from build123d import *

# Parameters (mm, degrees)
SKETCH1_R           = 54
SKETCH1_R_2         = 41
BOSS_EXTRUDE1_DEPTH = 10
SKETCH2_R           = 4.1
CUT_EXTRUDE1_DEPTH  = 5
CUT_EXTRUDE2_REACH  = 78.531
SKETCH3_R           = 3.1
CHAMFER1_SIZE       = 1


with BuildPart() as part:
    # Sketch1 → Boss-Extrude1 (new body)
    with BuildSketch(Plane(origin=(0, 0, 0), x_dir=(1, 0, 0), z_dir=(0, 1, 0))):
        with Locations(Location((0, 0, 0), (0, 0, 270))):
            Circle(SKETCH1_R)
        with Locations(Location((0, 0, 0), (0, 0, 270))):
            Circle(SKETCH1_R_2, mode=Mode.SUBTRACT)
    extrude(amount=BOSS_EXTRUDE1_DEPTH)

    # Sketch2 → Cut-Extrude1 (cut)
    with BuildSketch(Plane(origin=(0, 10, 0), x_dir=(1, 0, 0), z_dir=(0, 1, 0))):
        with Locations(Location((0, 47.5, 0), (0, 0, 270))):
            Circle(SKETCH2_R)
        with Locations(Location((41.13620668, -23.75, 0), (0, 0, 270))):
            Circle(SKETCH2_R)
        with Locations(Location((-41.13620668, -23.75, 0), (0, 0, 270))):
            Circle(SKETCH2_R)
    extrude(amount=-CUT_EXTRUDE1_DEPTH, mode=Mode.SUBTRACT)

    # Sketch3 → Cut-Extrude2 (cut, up to next)
    with BuildSketch(Plane(origin=(0, 5, 0), x_dir=(1, 0, 0), z_dir=(0, 1, 0)), mode=Mode.PRIVATE) as cut_extrude2_sk1:
        with Locations(Location((0, 47.5, 0), (0, 0, 270))):
            Circle(SKETCH3_R)
    cut_extrude2_tool1 = extrude(cut_extrude2_sk1.sketch, amount=-CUT_EXTRUDE2_REACH, mode=Mode.PRIVATE) & part.part
    # Sketch3 → Cut-Extrude2 (cut, up to next)
    with BuildSketch(Plane(origin=(0, 5, 0), x_dir=(1, 0, 0), z_dir=(0, 1, 0)), mode=Mode.PRIVATE) as cut_extrude2_sk2:
        with Locations(Location((41.13620668, -23.75, 0), (0, 0, 270))):
            Circle(SKETCH3_R)
    cut_extrude2_tool2 = extrude(cut_extrude2_sk2.sketch, amount=-CUT_EXTRUDE2_REACH, mode=Mode.PRIVATE) & part.part
    # Sketch3 → Cut-Extrude2 (cut, up to next)
    with BuildSketch(Plane(origin=(0, 5, 0), x_dir=(1, 0, 0), z_dir=(0, 1, 0)), mode=Mode.PRIVATE) as cut_extrude2_sk3:
        with Locations(Location((-41.13620668, -23.75, 0), (0, 0, 270))):
            Circle(SKETCH3_R)
    cut_extrude2_tool3 = extrude(cut_extrude2_sk3.sketch, amount=-CUT_EXTRUDE2_REACH, mode=Mode.PRIVATE) & part.part
    add(cut_extrude2_tool1.solids().sort_by_distance((0, 5, -47.5))[0], mode=Mode.SUBTRACT)
    add(cut_extrude2_tool2.solids().sort_by_distance((41.136207, 5, 23.75))[0], mode=Mode.SUBTRACT)
    add(cut_extrude2_tool3.solids().sort_by_distance((-41.136207, 5, 23.75))[0], mode=Mode.SUBTRACT)

    # Chamfer1
    chamfer1_edges = [part.edges().sort_by_distance(p)[0] for p in [
        (0, 10, -51.6),
        (41.13620668, 10, 19.65),
        (-41.13620668, 10, 19.65),
    ]]
    chamfer(chamfer1_edges, length=CHAMFER1_SIZE)


solid = part.part
Read the model definition and answer for the solid it produces. Units are mm, in the model's axes. A direction names the side the tool comes from. Coordinates: 2 decimals unless noted, no trailing zeros. Order: outer loops, then holes, each group sorted by start corner. A loop starts at its lowest first (then second) coordinate and runs counter-clockwise, first axis right, second up. Notation, with made-up numbers: (-11.75, 42.25) -> (18.25, 42.25) arc R16 cw to (18.25, 51.25) -> close; hole circle Ø7 at (3, 69.5). An arc over 180 degrees is marked (long way). Answer as a JSON object with one key per item and string values.
1) Each of these flat-tipped pins is pushed along its axis until it touches: pin 1 (10 mm diameter, centred on x = 41.14, z = 23.75, fed in from +Y); pin 2 (6.5 mm diameter, centred on x = 41, z = 25, fed in from +Y); pin 3 (5.5 mm diameter, centred on x = -41.14, z = 23.75, fed in from -Y); pin 4 (7 mm diameter, centred on x = 0, z = -47.5, fed in from +Y). Where does it stop, or does it pass through?
Model answer:
{"pin 1": "stops at y = 9.9", "pin 2": "stops at y = 9.41", "pin 3": "passes through", "pin 4": "stops at y = 5"}
2) A cutting plane is placed at C-C, the plane x = 20. Determine the outline of the cut face in (y, z), plus the area to 3 significant figures.
Model answer:
{"outline": "(0, -50.16) -> (10, -50.16) -> (10, -35.79) -> (0, -35.79) -> close; (0, 35.79) -> (10, 35.79) -> (10, 50.16) -> (0, 50.16) -> close", "area": "287 mm²"}
3) A cutting plane is placed at D-D, the plane z = 23.75. Determine the outline of the cut face in (x, y).
Model answer:
{"outline": "(-48.5, 0) -> (-44.24, 0) -> (-44.24, 5) -> (-45.24, 5) -> (-45.24, 9) -> (-46.24, 10) -> (-48.5, 10) -> close; (-38.04, 0) -> (-33.42, 0) -> (-33.42, 10) -> (-36.04, 10) -> (-37.04, 9) -> (-37.04, 5) -> (-38.04, 5) -> close; (33.42, 0) -> (38.04, 0) -> (38.04, 5) -> (37.04, 5) -> (37.04, 9) -> (36.04, 10) -> (33.42, 10) -> close; (44.24, 0) -> (48.5, 0) -> (48.5, 10) -> (46.24, 10) -> (45.24, 9) -> (45.24, 5) -> (44.24, 5) -> close"}
4) A tool of negligible diameter and unlimited length cuts with its end or side. For faces 4 (the face through (39.25, 2.54, 21.29)), 5 (the face through (43.91, 7.03, 20.73)), from which of +Z, -Z, +X, -X, +Y, -Y can it reach the whole face along a straight path? Write none if from no direction.
Model answer:
{"face 4": "+Y, -Y", "face 5": "+Y"}
5) The mould has two halves that part along X. Classify faces 1 (the face through (-36, 10, -20)), 2 (the face through (-1.187, 2.535, -44.636)), 3 (the face through (-52.716, 4.93, -11.706)): released by +X, released by -X, zero draft, split by the parting line, or undercut.
Model answer:
{"face 1": "zero draft", "face 2": "undercut", "face 3": "split by the parting line"}
6) Consider line 1 along X through (y, z) = (7, 0); line 2 along X through (y, z) = (3.5, 21); line 3 along X through (y, z) = (7.2, 23.75). Determine where each line is inside the solid, lowest interval first. Write a range as from..to.
Model answer:
{"line 1": "x = -54..-41, 41..54", "line 2": "x = -49.75..-42.57, -39.71..-35.21, 35.21..39.71, 42.57..49.75", "line 3": "x = -48.5..-45.24, -37.04..-33.42, 33.42..37.04, 45.24..48.5"}
7) A cutting plane is placed at B-B, the plane z = 0. Determine the outline of the cut face in (x, y), plus the area to 3 significant figures.
Model answer:
{"outline": "(-54, 0) -> (-41, 0) -> (-41, 10) -> (-54, 10) -> close; (41, 0) -> (54, 0) -> (54, 10) -> (41, 10) -> close", "area": "260 mm²"}
8) A cutting plane is placed at A-A, the plane x = 0. Determine the outline of the cut face in (y, z).
Model answer:
{"outline": "(0, -54) -> (10, -54) -> (10, -52.6) -> (9, -51.6) -> (5, -51.6) -> (5, -50.6) -> (0, -50.6) -> close; (0, -44.4) -> (5, -44.4) -> (5, -43.4) -> (9, -43.4) -> (10, -42.4) -> (10, -41) -> (0, -41) -> close; (0, 41) -> (10, 41) -> (10, 54) -> (0, 54) -> close"}
